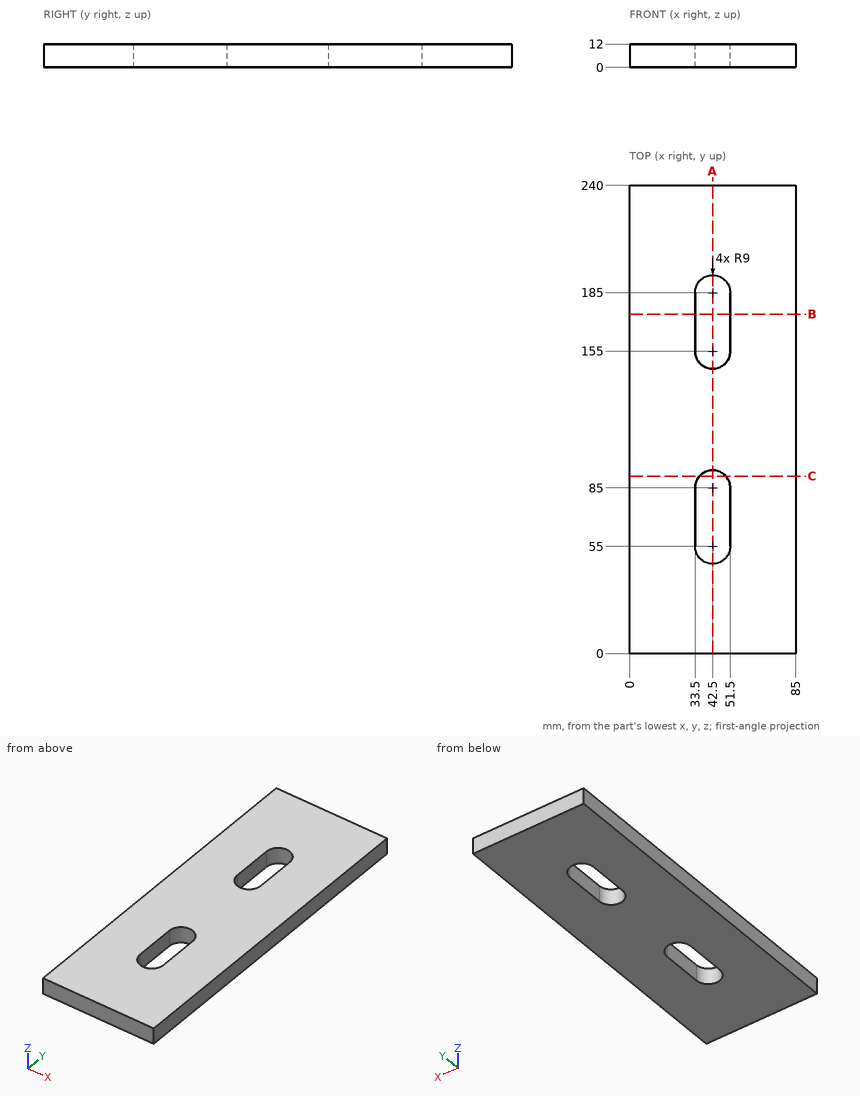
Print and shaded views of the part. All mm, measured from the part's lowest x, y and z. Round coordinates to 2 decimals unless told otherwise and drop trailing zeros. Order: outer loops, then holes, each group sorted by start corner. A loop starts at its lowest first (then second) coordinate and runs counter-clockwise, first axis right, second up. Notation, with made-up numbers: (76.5, 4) - (126.5, 4) arc R25 cw to (126.5, 23) - close; hole circle Ø11 at (70, 61.25). An arc over 180 degrees is marked (long way). Use a Markdown table: item, result.
1) Saw through at A-A on x = 42.5. Write the cut outline in (y, z), and give its area (3 significant figures).
Recorded:
| item | result |
|---|---|
| outline | (0, 0) - (46, 0) - (46, 12) - (0, 12) - close; (94, 0) - (146, 0) - (146, 12) - (94, 12) - close; (194, 0) - (240, 0) - (240, 12) - (194, 12) - close |
| area | 1,730 mm² |
2) Wall check: L1, parallel to X at y = 165.5, z = 5; L2, parallel to Y at x = 49, z = 2.25; L3, parallel to X at y = 188.5, z = 11.5. Give the ranges that are in metal, low to high.
Recorded:
| item | result |
|---|---|
| L1 | x = 0 to 33.5, 51.5 to 85 |
| L2 | y = 0 to 48.78, 91.22 to 148.78, 191.22 to 240 |
| L3 | x = 0 to 34.21, 50.79 to 85 |
3) Saw through at B-B on y = 174. Write the cut outline in (x, z).
Recorded:
| item | result |
|---|---|
| outline | (0, 0) - (33.5, 0) - (33.5, 12) - (0, 12) - close; (51.5, 0) - (85, 0) - (85, 12) - (51.5, 12) - close |
4) Saw through at C-C on y = 91. Write the cut outline in (x, z), and give its area (3 significant figures).
Recorded:
| item | result |
|---|---|
| outline | (0, 0) - (35.79, 0) - (35.79, 12) - (0, 12) - close; (49.21, 0) - (85, 0) - (85, 12) - (49.21, 12) - close |
| area | 859 mm² |
